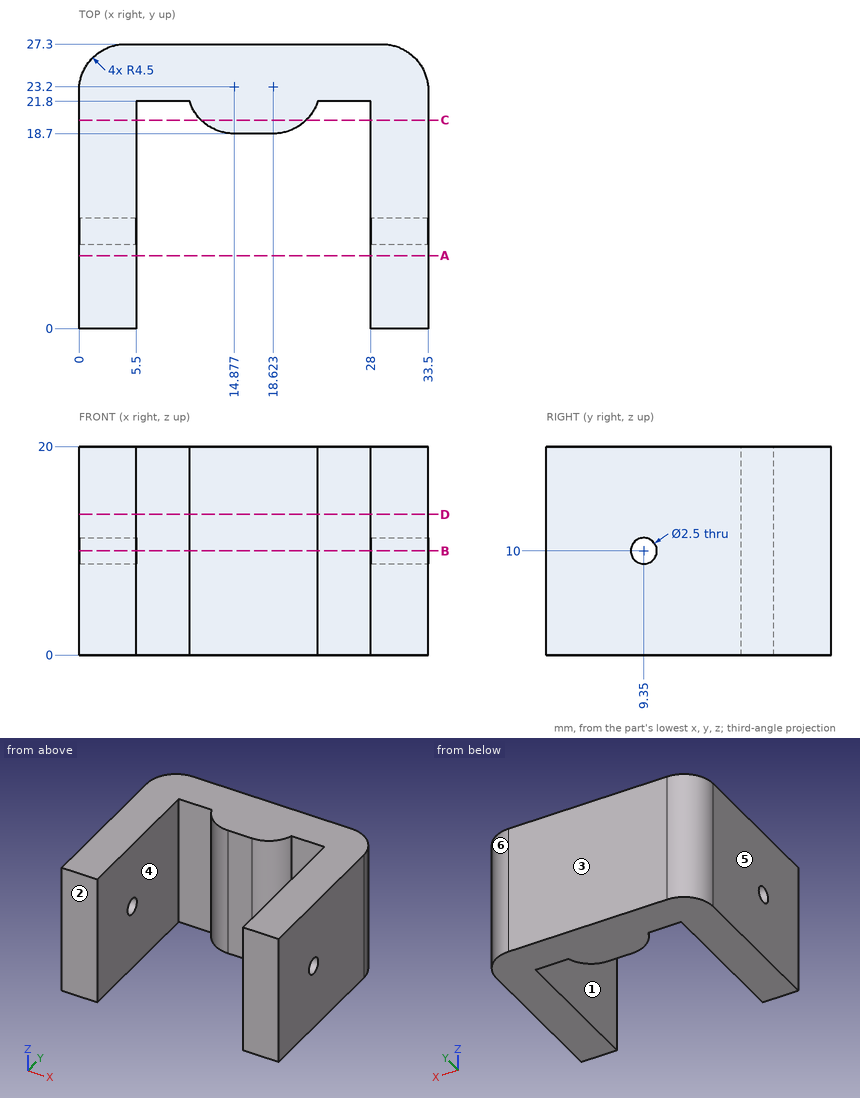
Design review of the part shown in the three views and the two pictorial views. Dimensions are in mm from the part's minimum x, y and z. A direction names the side the tool comes from. Round coordinates to 2 decimals unless told otherwise and drop trailing zeros. Loops run counter-clockwise (first coordinate to the right, second up) from the corner with the lowest first, then second, coordinate; pieces in that order, holes last. Notation, with made-up numbers: (49, -37.75) -> (73, -37.75) arc R36 cw to (73, 1.25) -> close; hole circle Ø3 at (52.5, 74). An arc over 180 degrees is marked (long way). Answer as a JSON object with one key per item and string values. Group by question number.
1) Mouldability with a two-part tool opening along X and no side actions: class the marked faces 3, 4, 5 and 6 as released by +X, released by -X, zero draft, split by the parting line, or undercut.
2) For pin 1 Ø2 at (x, z) = (23, 2) entering from -Y (1 decimal); pin 2 Ø1.5 at (y, z) = (9.35, 10) entering from +X; pin 3 Ø4 at (x, z) = (8, 12.5) entering from -Y; pin 4 Ø3 at (x, z) = (16, 8) entering from -Y, all flat-tipped, find the tip position at first contact; note any pin that passes through.
3) We need section D-D on z = 13.5. Write out the cut boundary in (x, y), then the cut area to 3 significant figures.
4) We need section C-C on y = 20. Write out the cut boundary in (x, z).
5) We need section A-A on y = 7. Write out the cut boundary in (x, z).
6) For the marked faces 1 and 2, list the 3-axis set-ups (+Z, -Z, +X, -X, +Y, -Y) from which the entire face can be reached by the end or side of a thin tool; tool diameter is ignored.
7) We need section B-B on z = 10. Write out the cut boundary in (x, y).
8) For line 1 (Z direction, x = 1.85, y = 9.35); line 2 (X direction, y = 3.25, z = 14); line 3 (Y direction, x = 8, z = 4.25), list the stretches that pass through material, from the lowest coordinate up. Write a range as [from, to].
Result set:
{
 "1": {"face 3": "zero draft", "face 4": "undercut", "face 5": "released by -X", "face 6": "released by +X"},
 "2": {"pin 1": "y = 20.2", "pin 2": "through", "pin 3": "y = 21.8", "pin 4": "y = 18.7"},
 "3": {"outline": "(0, 0) -> (5.5, 0) -> (5.5, 21.8) -> (10.6, 21.8) arc R4.5 ccw to (14.88, 18.7) -> (18.62, 18.7) arc R4.5 ccw to (22.9, 21.8) -> (28, 21.8) -> (28, 0) -> (33.5, 0) -> (33.5, 22.8) arc R4.5 ccw to (29, 27.3) -> (4.5, 27.3) arc R4.5 ccw to (0, 22.8) -> close", "area": "446 mm²"},
 "4": {"outline": "(0, 0) -> (5.5, 0) -> (5.5, 20) -> (0, 20) -> close; (11.71, 0) -> (21.79, 0) -> (21.79, 20) -> (11.71, 20) -> close; (28, 0) -> (33.5, 0) -> (33.5, 20) -> (28, 20) -> close"},
 "5": {"outline": "(0, 0) -> (5.5, 0) -> (5.5, 20) -> (0, 20) -> close; (28, 0) -> (33.5, 0) -> (33.5, 20) -> (28, 20) -> close"},
 "6": {"face 1": "+Z, -Z, -Y", "face 2": "+Z, -Z, +X, -X, -Y"},
 "7": {"outline": "(0, 0) -> (5.5, 0) -> (5.5, 8.1) -> (0, 8.1) -> close; (0, 10.6) -> (5.5, 10.6) -> (5.5, 21.8) -> (10.6, 21.8) arc R4.5 ccw to (14.88, 18.7) -> (18.62, 18.7) arc R4.5 ccw to (22.9, 21.8) -> (28, 21.8) -> (28, 10.6) -> (33.5, 10.6) -> (33.5, 22.8) arc R4.5 ccw to (29, 27.3) -> (4.5, 27.3) arc R4.5 ccw to (0, 22.8) -> close; (28, 0) -> (33.5, 0) -> (33.5, 8.1) -> (28, 8.1) -> close"},
 "8": {"line 1": "[0, 8.75], [11.25, 20]", "line 2": "[0, 5.5], [28, 33.5]", "line 3": "[21.8, 27.3]"}
}
